```python
from build123d import *

# Parameters (mm, degrees)
SKETCH1_R           = 10.287
BOSS_EXTRUDE1_DEPTH = 69.85
SKETCH2_W           = 16.51
SKETCH2_H           = 3.175
BOSS_EXTRUDE2_DEPTH = 20.6375
CUT_EXTRUDE1_DEPTH  = 92.841242236


with BuildPart() as part:
    # Sketch1 → Boss-Extrude1 (new body)
    with BuildSketch(Plane(origin=(0, 0, 0), x_dir=(1, 0, 0), z_dir=(0, 1, 0))):
        with Locations(Location((0, 0, 0), (0, 0, 270))):
            Circle(SKETCH1_R)
    extrude(amount=BOSS_EXTRUDE1_DEPTH)

    # Sketch2 → Boss-Extrude2 (add)
    with BuildSketch(Plane(origin=(0, 69.85, 0), x_dir=(1, 0, 0), z_dir=(0, 1, 0))):
        Rectangle(SKETCH2_W, SKETCH2_H)
    boss_extrude2 = extrude(amount=BOSS_EXTRUDE2_DEPTH)

    # Sketch3 → Cut-Extrude1 (cut, through all)
    with BuildSketch(Plane.XY.offset(1.5875)):
        with BuildLine():
            Line((3.7338, 82.0166), (3.7338, 76.8096))
            ThreePointArc((3.7338, 76.8096), (0, 73.0758), (-3.7338, 76.8096))
            Line((-3.7338, 76.8096), (-3.7338, 82.0166))
            ThreePointArc((-3.7338, 82.0166), (0, 85.7504), (3.7338, 82.0166))
        make_face()
    cut_extrude1 = extrude(amount=-CUT_EXTRUDE1_DEPTH, mode=Mode.SUBTRACT)

    # Mirror2: Boss-Extrude2, Cut-Extrude1 across plane
    add(boss_extrude2.mirror(Plane.ZX.offset(34.925)))
    add(cut_extrude1.mirror(Plane.ZX.offset(34.925)), mode=Mode.SUBTRACT)


solid = part.part
```
Geometry check sheet. Reference: the model listing, model coordinates, mm. A direction names the side the tool comes from. Coordinates: 2 decimals unless noted, no trailing zeros. Loops run counter-clockwise (first coordinate to the right, second up) from the corner with the lowest first, then second, coordinate; pieces in that order, holes last.
Item 1: Sectioned sample at A-A, the plane x = 0. Record the boundary of the cut face in (y, z).
Item 2: Sectioned sample at D-D, the plane y = 44. Record the boundary of the cut face in (x, z), then the cut area to 3 significant figures.
Item 3: Access from +Z, -Z, +X, -X, +Y, -Y to the whole of each face (thin tool, end or side, straight path). Record for faces 1 (the face through (8.255, 80, 0)), 2 (the face through (-4, -10, -1.588)), 3 (the face through (8.255, -10, 0)), 4 (the face through (-0.08, 85.75, 0.02)), 5 (the face through (-8.255, -10, 0)).
Item 4: Sectioned sample at C-C, the plane y = -10. Record the boundary of the cut face in (x, z) (1 decimal).
Item 5: Go/stop test with flat-tipped pins: pin 1 Ø1 at (y, z) = (80, 0) entering from +X (3 decimals); pin 2 Ø4 at (y, z) = (16.5, -5) entering from -X; pin 3 Ø3 at (x, y) = (-3.5, 7.5) entering from +Z; pin 4 Ø3 at (y, z) = (70, 0.5) entering from -X. Record where each tip stops, or that it passes through.
Item 6: Release check for a two-part mould opening along X. For faces 6 (the face through (0.082, 73.077, 0.022)), 7 (the face through (-4, 80, -1.588)), 8 (the face through (10.2, 34.44, -1.34)) record: released by +X, released by -X, zero draft, split by the parting line, or undercut.
Item 7: Sectioned sample at B-B, the plane z = 0. Count the separate pieces of the cut face and the enclosed holes in it, then the cut area to 3 significant figures.
Item 8: Thickness scan on line 1 (Y direction, x = 2.5, z = -1); line 2 (X direction, y = 33.5, z = -0.25); line 3 (Y direction, x = 6.5, z = -7.25). Record the ranges inside material, lowest first.
Check result:
1. outline: (-20.64, -1.59) - (-15.9, -1.59) - (-15.9, 1.59) - (-20.64, 1.59) - close; (-3.23, -1.59) - (0, -1.59) - (0, -10.29) - (69.85, -10.29) - (69.85, -1.59) - (73.08, -1.59) - (73.08, 1.59) - (69.85, 1.59) - (69.85, 10.29) - (0, 10.29) - (0, 1.59) - (-3.23, 1.59) - close; (85.75, -1.59) - (90.49, -1.59) - (90.49, 1.59) - (85.75, 1.59) - close
2. outline: circle Ø20.57 at (0, 0)
2. area: 332 mm2
3. face 1: +Z, -Z, +X, +Y
3. face 2: -Z, +X, -X, -Y
3. face 3: +Z, -Z, +X, -Y
3. face 4: +Z, -Z
3. face 5: +Z, -Z, -X, -Y
4. outline: (-8.3, -1.6) - (-3.7, -1.6) - (-3.7, 1.6) - (-8.3, 1.6) - close; (3.7, -1.6) - (8.3, -1.6) - (8.3, 1.6) - (3.7, 1.6) - close
5. pin 1: stops at x = 8.255
5. pin 2: stops at x = -9.84
5. pin 3: stops at z = 10.09
5. pin 4: stops at x = -10.29
6. face 6: undercut
6. face 7: zero draft
6. face 8: split by the parting line
7. separate pieces: 1
7. enclosed holes: 2
7. area: 1,950 mm2
8. line 1: y = -20.64 to -14.94, -4.19 to 74.04, 84.79 to 90.49
8. line 2: x = -10.28 to 10.28
8. line 3: y = 0 to 69.85
